from build123d import *

# Parameters (mm, degrees)
ESQUISSE1_R        = 2.75
BOSS_EXTRU_1_DEPTH = 1000


with BuildPart() as part:
    # Esquisse1 → Boss.-Extru.1 (new body)
    with BuildSketch(Plane(origin=(0, 0, 0), x_dir=(0, -1, 0), z_dir=(-1, 0, 0))):
        Polygon((-3, -10), (-3, -4.5), (3, -4.5), (3, -10), (10, -10), (10, -3), (4.5, -3), (4.5, 3), (10, 3), (10, 10), (3, 10), (3, 4.5), (-3, 4.5), (-3, 10), (-10, 10), (-10, 3), (-4.5, 3), (-4.5, -3), (-10, -3), (-10, -10), align=None)
        Circle(ESQUISSE1_R, mode=Mode.SUBTRACT)
    extrude(amount=-BOSS_EXTRU_1_DEPTH)


solid = part.part
Could you check a few things on this model? Use its own coordinates, in mm. Coordinates: 2 decimals unless noted, no trailing zeros. Write each loop counter-clockwise with the first axis right and the second up, starting at its lowest first coordinate (ties: lowest second). Pieces come first, ordered by that corner, then holes. Notation, with made-up numbers: (86.25, 11.25) - (143.25, 11.25) arc R24 cw to (143.25, 49.25) - close; hole circle Ø4 at (-33, -39). An arc over 180 degrees is marked (long way). Put each result on its own line as item: value. Start each with the question number.
Q1. Please list where these lines run through material, in increasing order: L1, parallel to Y at x = 547, z = 9.25; L2, parallel to Z at x = 579, y = 0.
Q2. I'm going to push flat-ended pins straight in: P1, Ø12, axis at y = 5.5, z = 8, coming from the -X side; P2, Ø3, axis at x = 456.5, z = 0.5, coming from the +Y side; P3, Ø1, axis at x = 814, z = -0.5, coming from the -Y side. Where does each tip first touch, or does it pass through?
Q3. I want a section at A-A on x = 122.5. Write out the boundary of the cut face in (y, z), plus the area to 3 significant figures.
Checks:
1. L1: -10 to -3, 3 to 10
1. L2: -4.5 to -2.75, 2.75 to 4.5
2. P1: x = 0
2. P2: y = 4.5
2. P3: y = -4.5
3. outline: (-10, -10) - (-3, -10) - (-3, -4.5) - (3, -4.5) - (3, -10) - (10, -10) - (10, -3) - (4.5, -3) - (4.5, 3) - (10, 3) - (10, 10) - (3, 10) - (3, 4.5) - (-3, 4.5) - (-3, 10) - (-10, 10) - (-10, 3) - (-4.5, 3) - (-4.5, -3) - (-10, -3) - close; hole circle Ø5.5 at (0, 0)
3. area: 244 mm²
